Autodesk Inventor part; units mm, degrees
ref_plane "YZ Plane" through (0, 0, 0) normal (1, 0, 0) x (0, 1, 0)
ref_plane "XZ Plane" through (0, 0, 0) normal (0, 1, 0) x (-1, 0, 0)
ref_plane "XY Plane" through (0, 0, 0) normal (0, 0, 1) x (1, 0, 0)
sketch "Sketch1" plane through (0, 0, 0) normal (0, 0, 1) x (1, 0, 0)
  line L0 (-13, 13) -> (13, 13) construction
  line L1 (13, 13) -> (13, -13) construction
  line L2 (13, -13) -> (-13, -13) construction
  line L3 (-13, -13) -> (-13, 13) construction
  circle A0 centre (-13, 13) radius 1.5
  circle A1 centre (-13, -13) radius 1.5
  circle A2 centre (-13, 13) radius 4
  circle A3 centre (-13, -13) radius 4
  line L4 (-15.7812, 15.8749) -> (-28.4765, 3.5936)
  arc A4 (-28.4765, 3.5936) -> (-28.4765, -3.5936) centre (-25, 0) ccw
  line L5 (-28.4765, -3.5936) -> (-15.7812, -15.8749)
  line L6 (-13, 17) -> (0, 17)
  line L7 (0, 17) -> (0, -17)
  line L8 (0, -17) -> (-13, -17)
  circle A5 centre (-25, 0) radius 3.25
  point P0 (0, 0)
  point P1 (0, 13)
  point P2 (-13, 0)
  point P3 (0, 0)
  dimension "d0" = 26
  dimension "d1" = 3
  dimension "d3" = 8
  dimension "d5" = 10
  dimension "d6" = 25
  dimension "d7" = 6.5
extrude "Extrusion1" add sketch "Sketch1" along normal blind 2
extrude "Extrusion2" add sketch "Sketch1" along normal blind 5 contours A2 | A3
mirror "Mirror1" about plane through (0, 0, 0) normal (1, 0, 0)
properties part number "adapter_board_mount"
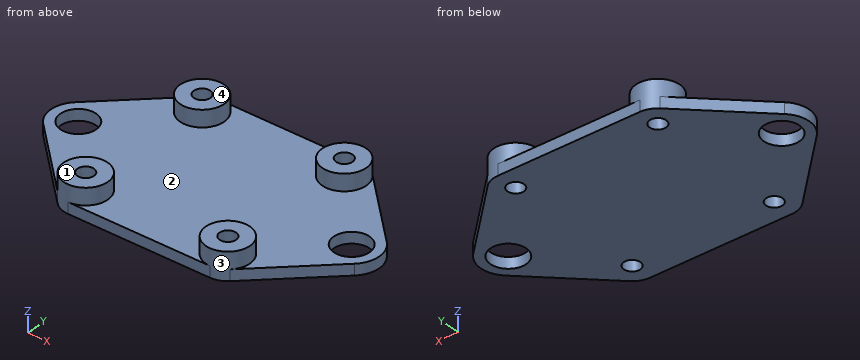
Part model, mm, in its own coordinate system. Face numbers are marked on the shaded views. A direction names the side the tool comes from. Give positions to 0.01 mm unless a question says otherwise; leave off trailing zeros. Write each loop counter-clockwise with the first axis right and the second up, starting at its lowest first coordinate (ties: lowest second). Pieces come first, ordered by that corner, then holes.
1) Cut at B-B on y = 0. Write the cut outline in (x, z).
Resolved:
outline: (-30, 0) - (-28.25, 0) - (-28.25, 2) - (-30, 2) - close; (-21.75, 0) - (21.75, 0) - (21.75, 2) - (-21.75, 2) - close; (28.25, 0) - (30, 0) - (30, 2) - (28.25, 2) - close
2) Which spindle directions (+Z, -Z, +X, -X, +Y, -Y) get a long thin tool onto all of the face, cutting with end or side? Do the marked faces 3 and 4. Say none if no direction does.
Resolved:
face 3: +Z
face 4: +Z, +X, -X, +Y, -Y
3) Pin check, flat tips, straight feed: pin 1 (3.5 mm diameter, centred on x = 13, y = 13, fed in from +Z); pin 2 (3 mm diameter, centred on x = -21, y = 4.5, fed in from +Z); pin 3 (1.5 mm diameter, centred on y = -7, z = 4, fed in from +X); pin 4 (3 mm diameter, centred on y = 8.5, z = 4, fed in from +X). Stop position of each tip, or through.
Resolved:
pin 1: stops at z = 5
pin 2: stops at z = 2
pin 3: passes through
pin 4: stops at x = 15.65
4) Cut at D-D on z = 0.6. Write the cut outline in (x, y), then the cut area to 3 significant figures.
Resolved:
outline: (-28.48, -3.59) - (-15.78, -15.87) arc R4 ccw to (-13, -17) - (13, -17) arc R4 ccw to (15.78, -15.87) - (28.48, -3.59) arc R5 ccw to (28.48, 3.59) - (15.78, 15.87) arc R4 ccw to (13, 17) - (-13, 17) arc R4 ccw to (-15.78, 15.87) - (-28.48, 3.59) arc R5 ccw to start; hole circle Ø6.5 at (-25, 0); hole circle Ø3 at (-13, -13); hole circle Ø3 at (-13, 13); hole circle Ø3 at (13, -13); hole circle Ø3 at (13, 13); hole circle Ø6.5 at (25, 0)
area: 1,480 mm2
5) Probe L1, parallel to Y at x = 13, z = 3.9; L2, parallel to Y at x = 13, z = 1.9; L3, parallel to Y at x = 14, z = 2.1. List the from-to ranges inside material, lowest first.
Resolved:
L1: y = -17 to -14.5, -11.5 to -9, 9 to 11.5, 14.5 to 17
L2: y = -17 to -14.5, -11.5 to 11.5, 14.5 to 17
L3: y = -16.87 to -14.12, -11.88 to -9.13, 9.13 to 11.88, 14.12 to 16.87
6) Two-plate mould, pull along X, no slides. Class the marked faces 1 and 2: released by +X, released by -X, zero draft, split by the parting line, or undercut.
Resolved:
face 1: zero draft
face 2: undercut
7) Cut at C-C on x = -25. Write the cut outline in (y, z).
Resolved:
outline: (-6.96, 0) - (-3.25, 0) - (-3.25, 2) - (-6.96, 2) - close; (3.25, 0) - (6.96, 0) - (6.96, 2) - (3.25, 2) - close
8) Cut at A-A on z = 3.35. Write the cut outline in (x, y).
Resolved:
outline: circle Ø8 at (-13, -13); circle Ø8 at (-13, 13); circle Ø8 at (13, -13); circle Ø8 at (13, 13); hole circle Ø3 at (-13, -13); hole circle Ø3 at (-13, 13); hole circle Ø3 at (13, -13); hole circle Ø3 at (13, 13)
